```python
from build123d import *

# Parameters (mm, degrees)
F1_DEPTH = 300
F2_R     = 120
F3_DEPTH = 270
F4_W     = 308.2067033212
F4_H     = 85.1061673835
F4_H_2   = 71.9743549824
F5_DEPTH = 160
F6_W     = 120
F6_H     = 100
F7_DEPTH = 100
F8_W     = 60
F8_H     = 40
F9_DEPTH = 450.001


with BuildPart() as f1:
    # F0 (on Front) → F1 (new body)
    with BuildSketch(Plane.XZ):
        Polygon((-225, -9.4181643799), (-225, -75), (225, -75), (225, -9.4181643799), (120, 75), (-120, 75), align=None)
    extrude(amount=F1_DEPTH)

    # F2 (on face) → F3 (join)
    with BuildSketch(Plane.XY.offset(75)):
        with Locations((0, -150)):
            Circle(F2_R)
    extrude(amount=F3_DEPTH)

    # F4 (on face) → F5 (cut)
    with BuildSketch(Plane.XY.offset(345)):
        with Locations((0, -57.4469163083)):
            Rectangle(F4_W, F4_H)
        with Locations((0, -235.9871774912)):
            Rectangle(F4_W, F4_H_2)
    extrude(amount=-F5_DEPTH, mode=Mode.SUBTRACT)

    # F6 (on face) → F7 (cut)
    with BuildSketch(Plane.XY.offset(345)):
        with Locations((0, -150)):
            Rectangle(F6_W, F6_H)
    extrude(amount=-F7_DEPTH, mode=Mode.SUBTRACT)

    # F8 (on face) → F9 (cut, through all)
    with BuildSketch(Plane(origin=(-225, 0, 0), x_dir=(0, -1, 0), z_dir=(-1, 0, 0))):
        with Locations((150, -75)):
            Rectangle(F8_W, F8_H)
        Polygon((75, 0), (120, -55), (180, -55), (225, 0), (225, 30), (75, 30), align=None)
    extrude(amount=-F9_DEPTH, mode=Mode.SUBTRACT)


solid = f1.part
```
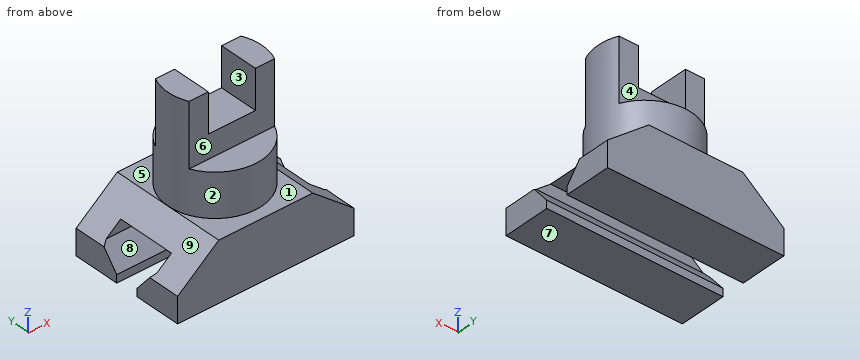
Input: part model. Units: mm. Frame: model coordinates. Face numbers are marked on the shaded views. A direction names the side the tool comes from. Give positions to 0.01 mm unless a question says otherwise; leave off trailing zeros. Order: outer loops, then holes, each group sorted by start corner. A loop starts at its lowest first (then second) coordinate and runs counter-clockwise, first axis right, second up. Notation, with made-up numbers: M 88,-12 L 133,-12 A26 ccw 133,13 Z; hole C 43,87.5 d5. An arc over 180 degrees is marked long. Return JSON: item names as keys, results as strings.
1) Section query A-A on x = 0. Output: boundary loops of the cut face in (y, z).
Taken from the geometry:
{"outline": "M -300,-75 L -180,-75 L -180,-55 L -225,0 L -225,30 L -75,30 L -75,0 L -120,-55 L -120,-75 L 0,-75 L 0,75 L -30,75 L -30,185 L -100,185 L -100,245 L -200,245 L -200,185 L -270,185 L -270,75 L -300,75 Z"}
2) Section query C-C on z = 206. Output: boundary loops of the cut face in (x, y), and give its area (3 significant figures).
Taken from the geometry:
{"outline": "M -109.09,-200 L 109.09,-200 A120 ccw 109.09,-100 L -109.09,-100 A120 ccw Z", "area": "23,300 mm2"}
3) Contact query for flat-ended pins moving along their axis: pin 1 (12 mm diameter, centred on y = -189.5, z = 222.5, fed in from +X); pin 2 (6 mm diameter, centred on x = -52.5, z = 84.5, fed in from +Y); pin 3 (4 mm diameter, centred on x = 3.5, y = -256.5, fed in from +Z); pin 4 (16 mm diameter, centred on x = -83.5, z = -68.5, fed in from +Y). Output: stop coordinate, or through.
Taken from the geometry:
{"pin 1": "stops at x = 115.23", "pin 2": "stops at y = -40.69", "pin 3": "stops at z = 185", "pin 4": "stops at y = 0"}
4) Mould query, pull axis Z, two halves, no side actions, for the marked faces 6, 7, 8 and 9. Classes: released by +Z, released by -Z, zero draft, split by the parting line, or undercut.
Taken from the geometry:
{"face 6": "zero draft", "face 7": "released by -Z", "face 8": "undercut", "face 9": "released by +Z"}
5) Section query D-D on y = -259. Output: boundary loops of the cut face in (x, z), and give its area (3 significant figures).
Taken from the geometry:
{"outline": "M -225,-75 L 225,-75 L 225,-9.42 L 120,75 L 50.19,75 L 50.19,185 L -50.19,185 L -50.19,75 L -120,75 L -225,-9.42 Z", "area": "69,700 mm2"}
6) Access query for the marked faces 1, 2, 3, 4 and 5. Directions: +Z, -Z, +X, -X, +Y, -Y. A direction counts if a zero-diameter tool reaches every point of the face in a straight line with its end or side. Return the directions, or none.
Taken from the geometry:
{"face 1": "+Z, -Y", "face 2": "+Z", "face 3": "+Z, +Y, -Y", "face 4": "+Z, +X, -X, +Y", "face 5": "+Z, +Y"}
7) Section query B-B on y = -209.5. Output: boundary loops of the cut face in (x, z), and give its area (3 significant figures).
Taken from the geometry:
{"outline": "M -225,-75 L 225,-75 L 225,-18.94 L -225,-18.94 Z; M -175.97,30 L 175.97,30 L 120,75 L 104.21,75 L 104.21,185 L -104.21,185 L -104.21,75 L -120,75 Z", "area": "61,500 mm2"}
8) Line query: L1, parallel to Z at x = 79, y = -125; L2, parallel to Z at x = -22, y = -230.5; L3, parallel to Y at x = -160.5, z = -7. Output: solid intervals per line, ascending. Write a range as [from, to].
Taken from the geometry:
{"L1": "z = [30, 345]", "L2": "z = [-75, 185]", "L3": "y = [-300, -219.27], [-80.73, 0]"}
